Source: CAD feature listing. Evaluate the final solid. Frame: model axes, mm. Face numbers are marked on the shaded views. A direction names the side the tool comes from. Give positions to 0.01 mm unless a question says otherwise; leave off trailing zeros. Order: outer loops, then holes, each group sorted by start corner. A loop starts at its lowest first (then second) coordinate and runs counter-clockwise, first axis right, second up.
from build123d import *

# Parameters (mm, degrees)
BOSS_EXTRUDE1_DEPTH     = 127
FILLET1_R               = 2.54
BOSS_EXTRUDE2_DEPTH     = 38.1
CUT_EXTRUDE1_DEPTH      = 176.221279464
CUT_EXTRUDE1_DEPTH_BACK = 176.221279464
SKETCH4_R               = 3.675
FILLET2_R               = 1
FILLET3_R               = 6.35


with BuildPart() as part:
    # Sketch1 → Boss-Extrude1 (new body)
    with BuildSketch(Plane.XY):
        with BuildLine():
            Line((-71.414284285, -70), (71.414284285, -70))
            ThreePointArc((71.414284285, -70), (0, -100), (-71.414284285, -70))
        make_face()
    extrude(amount=BOSS_EXTRUDE1_DEPTH)

    # Fillet1
    fillet1_edges = [part.edges().sort_by_distance(p)[0] for p in [
        (-71.414284285, -70, 63.5),
        (71.414284285, -70, 63.5),
    ]]
    fillet(fillet1_edges, radius=FILLET1_R)

    # Sketch2 → Boss-Extrude2 (add)
    with BuildSketch(Plane(origin=(0, -70, 0), x_dir=(1, 0, 0), z_dir=(0, 1, 0))):
        Polygon((-58.737633234, -6.35), (-58.737633234, 0), (-43.815133234, 0), (-43.815133234, -25.4), (-58.737633234, -25.4), (-58.737633234, -19.05), (-55.562633234, -19.05), (-55.562633234, -22.225), (-53.340133234, -22.225), (-46.990133234, -12.7), (-53.340133234, -3.175), (-55.562633234, -3.175), (-55.562633234, -6.35), align=None)
    boss_extrude2 = extrude(amount=BOSS_EXTRUDE2_DEPTH)

    # Mirror1: Boss-Extrude2 across plane
    add(boss_extrude2.mirror(Plane(origin=(0, 0, 0), x_dir=(0, 0, 1), z_dir=(1, 0, 0))))

    # Sketch4 → Cut-Extrude1 (cut, two sides: drawn at the far end of the back side and taken through both)
    with BuildSketch(Plane(origin=(0, 0, 0), x_dir=(0, 0, -1), z_dir=(1, 0, 0)).offset(-CUT_EXTRUDE1_DEPTH_BACK)):
        with Locations(Location((-12.7, -38.25, 0), (0, 0, 270))):
            Circle(SKETCH4_R)
    extrude(amount=CUT_EXTRUDE1_DEPTH + CUT_EXTRUDE1_DEPTH_BACK, mode=Mode.SUBTRACT)

    # Fillet2
    # the kernel refuses this fillet: 1 mm, written as the material it adds along each edge
    with BuildSketch(Plane(origin=(55.562633234, -72.5, 3.175), x_dir=(-1, 0, 0), z_dir=(0, 1, 0)), Plane(origin=(55.562633234, -72.5, 22.225), x_dir=(0, 0, -1), z_dir=(0, 1, 0)), Plane(origin=(-55.562633234, -72.5, 22.225), x_dir=(1, 0, 0), z_dir=(0, 1, 0)), Plane(origin=(-55.562633234, -72.5, 3.175), x_dir=(0, 0, 1), z_dir=(0, 1, 0))) as fillet2_piece_1:
        with BuildLine():
            CenterArc((FILLET2_R, FILLET2_R), FILLET2_R, 180, 90)
            Line((0, FILLET2_R), (0, 0))
            Line((0, 0), (FILLET2_R, 0))
        make_face()
    extrude(amount=40.6)
    with BuildSketch(Plane(origin=(53.340133234, -71.337959396, 3.175), x_dir=(-0.5547001962252287, 0, 0.8320502943378439), z_dir=(0, 1, 0)), Plane(origin=(53.340133234, -71.337959396, 22.225), x_dir=(1, 0, 0), z_dir=(0, 1, 0)), Plane(origin=(-53.340133234, -71.337959396, 22.225), x_dir=(0.5547001962252323, 0, -0.8320502943378416), z_dir=(0, 1, 0)), Plane(origin=(-53.340133234, -71.337959396, 3.175), x_dir=(-1, 0, 0), z_dir=(0, 1, 0))) as fillet2_piece_2:
        with BuildLine():
            CenterArc((FILLET2_R * 0.535183758488, FILLET2_R), FILLET2_R, 213.690067526, 56.309932474)
            Line((-FILLET2_R * 0.29686653585, FILLET2_R * 0.445299803775), (0, 0))
            Line((0, 0), (FILLET2_R * 0.535183758488, 0))
        make_face()
    extrude(amount=39.437959396)
    with BuildSketch(Plane(origin=(46.990133234, -36.241666667, 12.7), x_dir=(0.5547001962252254, 0, 0.832050294337846), z_dir=(0, 1, 0))) as fillet2_piece_3_section:
        with BuildLine():
            CenterArc((FILLET2_R * 0.666666666667, FILLET2_R), FILLET2_R, 202.619864948, 67.380135052)
            Line((-FILLET2_R * 0.25641025641, FILLET2_R * 0.615384615385), (0, 0))
            Line((0, 0), (FILLET2_R * 0.666666666667, 0))
        make_face()
    fillet2_piece_3 = extrude(amount=4.341666667, mode=Mode.PRIVATE)
    fillet2_piece_3 = fillet2_piece_3 - Plane(origin=(47.151998472, -38.25, 12.7), x_dir=(0, -1, 0), z_dir=(-1, 0, 0)) * Cylinder(3.675, 12, mode=Mode.PRIVATE)
    add(fillet2_piece_3)
    with BuildSketch(Plane(origin=(46.990133234, -71.666666667, 12.7), x_dir=(0.554700196225229, 0, 0.8320502943378436), z_dir=(0, 1, 0))) as fillet2_piece_4_section:
        with BuildLine():
            CenterArc((FILLET2_R * 0.666666666667, FILLET2_R), FILLET2_R, 202.619864948, 67.380135052)
            Line((-FILLET2_R * 0.25641025641, FILLET2_R * 0.615384615385), (0, 0))
            Line((0, 0), (FILLET2_R * 0.666666666667, 0))
        make_face()
    fillet2_piece_4 = extrude(amount=31.408333333, mode=Mode.PRIVATE)
    fillet2_piece_4 = fillet2_piece_4 - Plane(origin=(47.151783085, -38.25, 12.7), x_dir=(0, -1, 0), z_dir=(-1, 0, 0)) * Cylinder(3.675, 66, mode=Mode.PRIVATE)
    add(fillet2_piece_4)
    with BuildSketch(Plane(origin=(-46.990133234, -71.666666667, 12.7), x_dir=(-0.5547001962252304, 0, -0.8320502943378429), z_dir=(0, 1, 0))) as fillet2_piece_5_section:
        with BuildLine():
            CenterArc((FILLET2_R * 0.666666666667, FILLET2_R), FILLET2_R, 202.619864948, 67.380135052)
            Line((-FILLET2_R * 0.25641025641, FILLET2_R * 0.615384615385), (0, 0))
            Line((0, 0), (FILLET2_R * 0.666666666667, 0))
        make_face()
    fillet2_piece_5 = extrude(amount=31.408333333, mode=Mode.PRIVATE)
    fillet2_piece_5 = fillet2_piece_5 - Plane(origin=(-47.151783085, -38.25, 12.7), x_dir=(0, -1, 0), z_dir=(1, 0, 0)) * Cylinder(3.675, 66, mode=Mode.PRIVATE)
    add(fillet2_piece_5)
    with BuildSketch(Plane(origin=(-46.990133234, -36.241666667, 12.7), x_dir=(-0.554700196225229, 0, -0.8320502943378436), z_dir=(0, 1, 0))) as fillet2_piece_6_section:
        with BuildLine():
            CenterArc((FILLET2_R * 0.666666666667, FILLET2_R), FILLET2_R, 202.619864948, 67.380135052)
            Line((-FILLET2_R * 0.25641025641, FILLET2_R * 0.615384615385), (0, 0))
            Line((0, 0), (FILLET2_R * 0.666666666667, 0))
        make_face()
    fillet2_piece_6 = extrude(amount=4.341666667, mode=Mode.PRIVATE)
    fillet2_piece_6 = fillet2_piece_6 - Plane(origin=(-47.151998479, -38.25, 12.7), x_dir=(0, -1, 0), z_dir=(1, 0, 0)) * Cylinder(3.675, 12, mode=Mode.PRIVATE)
    add(fillet2_piece_6)
    # the kernel refuses this fillet: 1 mm, written as the material it takes off along each edge
    with BuildSketch(Plane(origin=(55.562633234, -70, 19.05), x_dir=(0, 0, 1), z_dir=(0, 1, 0)), Plane(origin=(55.562633234, -70, 6.35), x_dir=(1, 0, 0), z_dir=(0, 1, 0)), Plane(origin=(-55.562633234, -70, 19.05), x_dir=(-1, 0, 0), z_dir=(0, 1, 0)), Plane(origin=(-55.562633234, -70, 6.35), x_dir=(0, 0, -1), z_dir=(0, 1, 0))) as fillet2_2_piece_1:
        with BuildLine():
            CenterArc((FILLET2_R, FILLET2_R), FILLET2_R, 180, 90)
            Line((0, FILLET2_R), (0, 0))
            Line((0, 0), (FILLET2_R, 0))
        make_face()
    extrude(amount=40.6, mode=Mode.SUBTRACT)

    # Fillet3
    fillet3_edges = [part.edges().sort_by_distance(p)[0] for p in [
        (-43.815133234, -50.95, 25.4),
        (-43.815133234, -50.95, 0),
        (43.815133234, -50.95, 0),
        (43.815133234, -50.95, 25.4),
    ]]
    fillet(fillet3_edges, radius=FILLET3_R)


solid = part.part
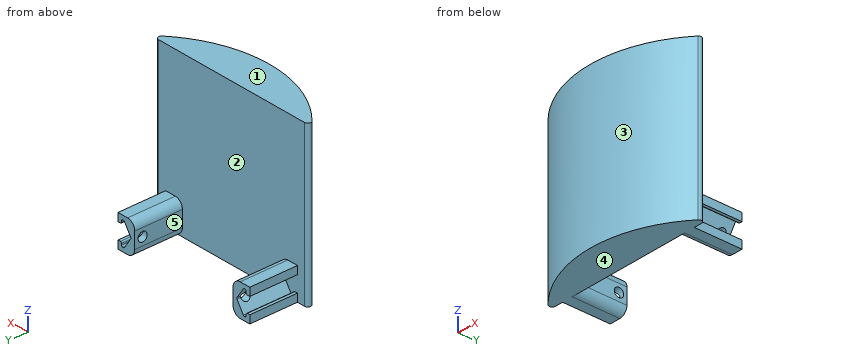
(1) Pin query (flat end, axial travel): pin 1 Ø1 at (y, z) = (-86.5, 61.5) entering from -X; pin 2 Ø6 at (y, z) = (-79.5, 111) entering from +X; pin 3 Ø7 at (y, z) = (-53.5, 3) entering from +X. Return the tip coordinate at first contact, or that it passes through.
(2) Draft query along X for the marked faces 1, 2 and 3. Return one class per face: +X half, -X half, draft (parallel to the pull), parting line (faces both ways), or undercut.
(3) Access query for the marked faces 4 and 5. Directions: +Z, -Z, +X, -X, +Y, -Y. A direction counts if a zero-diameter tool reaches every point of the face in a straight line with its end or side. Return the directions, or none.
(4) Section B-B, the plane z = 53.5. Return loops of the section in (x, y), plus the area to 3 significant figures.
(5) Line query: line 1 along Z through (x, y) = (-47, -38); line 2 along Z through (x, y) = (-44.5, -39); line 3 along Y through (x, z) = (41, 73). Output: solid intervals per line, ascending.
(6) Section A-A, the plane x = 2. Return loops of the section in (y, z).
Checks:
1. pin 1: stops at x = -51.03
1. pin 2: stops at x = 64.4
1. pin 3: stops at x = 58.74
2. face 1: draft
2. face 2: undercut
2. face 3: parting line
3. face 4: -Z, +X, -X, +Y, -Y
3. face 5: +Z, -Z, +Y
4. outline: (-66.78, -74.43) arc R100 ccw to (66.78, -74.43) arc R2.54 ccw to (65.09, -70) - (-65.09, -70) arc R2.54 ccw to start
4. area: 2,940 mm2
5. line 1: z = 0.85 to 9.03, 16.37 to 24.55
5. line 2: z = 3.48 to 9.1, 16.3 to 21.92
5. line 3: y = -91.21 to -70
6. outline: (-99.98, 0) - (-70, 0) - (-70, 127) - (-99.98, 127) - close
